Geometry: see drawing. Coordinates: mm, zero at the bounding-box minimum. A direction names the side the tool comes from. Coordinates: 2 decimals unless noted, no trailing zeros. Write each loop counter-clockwise with the first axis right and the second up, starting at its lowest first coordinate (ties: lowest second). Pieces come first, ordered by that corner, then holes. Notation, with made-up numbers: (82.25, 5.5) - (88.25, 5.5) arc R16 cw to (88.25, 15.5) - close; hole circle Ø5 at (39.25, 56). An arc over 180 degrees is marked (long way). One line per question, with ' | ' between items. Start each with the question number.
1) Reachability of the marked faces 1, 2, 3, 4 and 5 from +Z, -Z, +X, -X, +Y, -Y: full face, straight path, thin tool, end or side. Return the list, or none.
2) Line query: line 1 (X direction, y = 1.75, z = 13.5); line 2 (Y direction, x = 11.75, z = 5.5); line 3 (X direction, y = 2.25, z = 14.25). Output: solid intervals per line, ascending.
3) Section query B-B on y = 11.4. Return loops of the section in (x, z), and give its area (3 significant figures).
4) Section query A-A on z = 13.5. Return loops of the section in (x, y), and give its area (3 significant figures).
5) Section query C-C on x = 18. Return loops of the section in (y, z), and give its area (3 significant figures).
6) Draft query along Z for the marked faces 6, 7 and 8. Return one class per face: released by +Z, released by -Z, zero draft, split by the parting line, or undercut.
7) First-contact query: P1, Ø6, axis at y = 9, z = 6.5, coming from the +X side; P2, Ø4, axis at y = 11.5, z = 11.5, coming from the -X side; P3, Ø5.5, axis at x = 7, y = 2, coming from the -Z side; P4, Ø4, axis at x = 18, z = 13.5, coming from the -Y side. Flat tips, straight axial feed; report the tip coordinate or a pass-through.
8) Section query D-D on x = 11. Return loops of the section in (y, z), and give its area (3 significant figures).
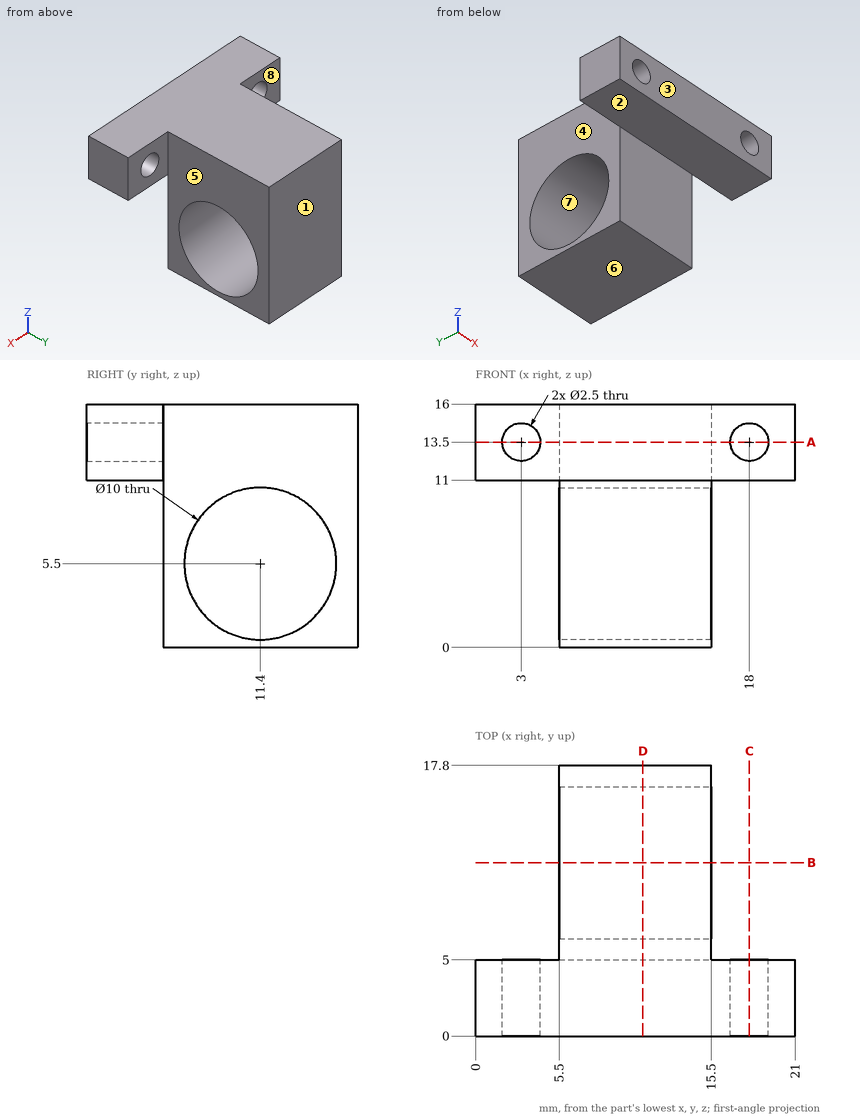
Answer key:
1) face 1: +Z, -Z, +X, -X, +Y | face 2: -Z, +X, -X, -Y | face 3: +Z, -Z, +X, -X, -Y | face 4: +Z, -Z, -X, +Y | face 5: +Z, -Z, +X, +Y
2) line 1: 0 to 1.75, 4.25 to 16.75, 19.25 to 21 | line 2: 5 to 6.4, 16.4 to 17.8 | line 3: 0 to 2, 4 to 17, 19 to 21
3) outline: (5.5, 0) - (15.5, 0) - (15.5, 0.5) - (5.5, 0.5) - close; (5.5, 10.5) - (15.5, 10.5) - (15.5, 16) - (5.5, 16) - close | area: 60.0 mm²
4) outline: (0, 0) - (1.75, 0) - (1.75, 5) - (0, 5) - close; (4.25, 0) - (16.75, 0) - (16.75, 5) - (15.5, 5) - (15.5, 17.8) - (5.5, 17.8) - (5.5, 5) - (4.25, 5) - close; (19.25, 0) - (21, 0) - (21, 5) - (19.25, 5) - close | area: 208 mm²
5) outline: (0, 11) - (5, 11) - (5, 12.25) - (0, 12.25) - close; (0, 14.75) - (5, 14.75) - (5, 16) - (0, 16) - close | area: 12.5 mm²
6) face 6: released by -Z | face 7: undercut | face 8: zero draft
7) P1: x = 15.5 | P2: x = 5.5 | P3: z = 11 | P4: y = 0
8) outline: (0, 11) - (5, 11) - (5, 0) - (17.8, 0) - (17.8, 16) - (0, 16) - close; hole circle Ø10 at (11.4, 5.5) | area: 151 mm²
